Autodesk Inventor part; units mm, degrees
ref_plane "YZ Plane" through (0, 0, 0) normal (1, 0, 0) x (0, 1, 0)
ref_plane "XZ Plane" through (0, 0, 0) normal (0, 1, 0) x (-1, 0, 0)
ref_plane "Work Plane1" through (0, 0, -20) normal (0, 0, 1) x (1, 0, 0)
sketch "Sketch1" plane through (0, 0, -20) normal (0, 0, 1) x (1, 0, 0)
  circle A0 centre (-1.75, 0) radius 15.5
  circle A1 centre (-1.75, 0) radius 7.5
  point P0 (0, 0)
  dimension "d1" = 15
extrude "Extrusion1" add sketch "Sketch1" along normal blind 1 contours A1
sketch "Sketch2" plane through (-1.75, 0, -19) normal (0, 0, 1) x (1, 0, 0)
  circle A0 centre (0, 0) radius 7.5
  circle A1 centre (0, 0) radius 6
  point P0 (1.75, 0)
  dimension "d4" = 12
extrude "Extrusion2" add sketch "Sketch2" along normal blind 8 contours A1
sketch "Sketch3" plane through (-1.75, 0, -11) normal (0, 0, 1) x (1, 0, 0)
  circle A0 centre (0, 0) radius 7.5
  circle A1 centre (0, 0) radius 7.5
  point P0 (1.75, 0)
extrude "Extrusion3" add sketch "Sketch3" along normal blind 7
properties part number "small pulley"
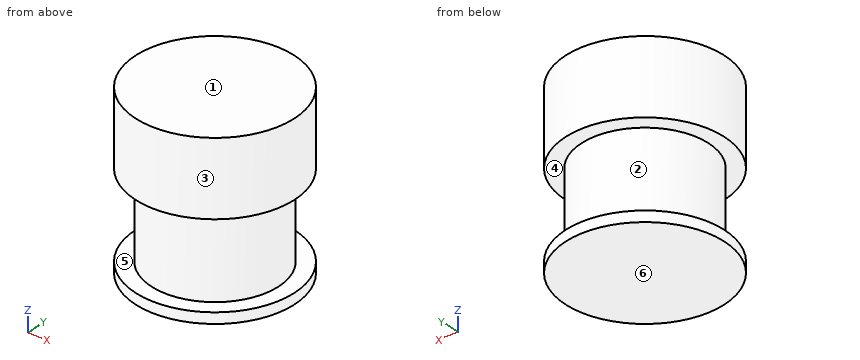
The model under review builds one solid part; all positions refer to its coordinate system, in mm. Face numbers are marked on the shaded views. A direction names the side the tool comes from. Round coordinates to 2 decimals unless told otherwise and drop trailing zeros. Loops run counter-clockwise (first coordinate to the right, second up) from the corner with the lowest first, then second, coordinate; pieces in that order, holes last. Notation, with made-up numbers: (86.25, -23) -> (107.25, -23) arc R22 cw to (107.25, 2) -> close; hole circle Ø10 at (46, 86.5). An arc over 180 degrees is marked (long way). Answer as CSV lines item,"result".
1) Tool access review of the marked faces 5 and 6: name each direction out of +Z, -Z, +X, -X, +Y, -Y from which nothing blocks a thin tool from reaching the whole face with its end or side.
Geometry results:
face 5,"none"
face 6,"-Z, +X, -X, +Y, -Y"
2) For P1, Ø8, axis at x = -6.5, z = -6.5, coming from the +Y side; P2, Ø6, axis at y = -3.5, z = -10, coming from the -X side; P3, Ø2, axis at x = -5, z = -14, coming from the -Y side, all flat-tipped, find the tip position at first contact; note any pin that passes through.
Geometry results:
P1,"stops at y = 7.46"
P2,"stops at x = -9.23"
P3,"stops at y = -5.56"
3) Add section D-D on y = 0. Write out the cut boundary in (x, z), plus the area to 3 significant figures.
Geometry results:
outline,"(-9.25, -20) -> (5.75, -20) -> (5.75, -19) -> (4.25, -19) -> (4.25, -11) -> (5.75, -11) -> (5.75, -4) -> (-9.25, -4) -> (-9.25, -11) -> (-7.75, -11) -> (-7.75, -19) -> (-9.25, -19) -> close"
area,"216 mm²"
4) Add section C-C on z = -9.25. Write out the cut boundary in (x, y).
Geometry results:
outline,"circle Ø15 at (-1.75, 0)"
5) Draft analysis for pull direction Z (two halves, no side actions). For the marked faces 1, 2, 3 and 4, state which applies: pulls with the +Z half, pulls with the -Z half, needs draft (parallel to the pull), parting line crosses it, or undercut.
Geometry results:
face 1,"pulls with the +Z half"
face 2,"undercut"
face 3,"needs draft"
face 4,"undercut"
6) Add section A-A on y = 6.5. Write out the cut boundary in (x, z).
Geometry results:
outline,"(-5.49, -20) -> (1.99, -20) -> (1.99, -19) -> (-5.49, -19) -> close; (-5.49, -11) -> (1.99, -11) -> (1.99, -4) -> (-5.49, -4) -> close"
7) Add section B-B on x = -1.75. Write out the cut boundary in (y, z), plus the area to 3 significant figures.
Geometry results:
outline,"(-7.5, -20) -> (7.5, -20) -> (7.5, -19) -> (6, -19) -> (6, -11) -> (7.5, -11) -> (7.5, -4) -> (-7.5, -4) -> (-7.5, -11) -> (-6, -11) -> (-6, -19) -> (-7.5, -19) -> close"
area,"216 mm²"
8) To check wall thickness, follow line 1 along Z through (x, y) = (-8.5, -0.75); line 2 along Y through (x, z) = (2, -14.25); line 3 along X through (y, z) = (-0.25, -7). State the ranges of each line that lie inside material, in increasing order. Write a range as from..to.
Geometry results:
line 1,"z = -20..-19, -11..-4"
line 2,"y = -4.68..4.68"
line 3,"x = -9.25..5.75"
